The listing builds one solid part. Answer for the finished solid, in the listing's coordinates (mm). Face numbers are marked on the shaded views. A direction names the side the tool comes from. Coordinates: 2 decimals unless noted, no trailing zeros. Loops run counter-clockwise (first coordinate to the right, second up) from the corner with the lowest first, then second, coordinate; pieces in that order, holes last. Notation, with made-up numbers: M 11,61.5 L 50,61.5 A27 cw 50,79.5 Z; hole C -32,11.5 d11. An arc over 180 degrees is marked long. Answer as a JSON object with one key per item and string values. Group by question number.
1. Straight lines are drawn through the part: L1, parallel to Z at x = 18, y = -8.5; L2, parallel to Z at x = -9, y = 3; L3, parallel to X at y = 0.75, z = -3.5. For each, find the intervals that lie inside material, in ascending order.
2. A cutting plane is placed at D-D on z = -3.5. Give the vertices of the cut face in (x, y).
3. A cutting plane is placed at A-A on x = 41. Give the vertices of the cut face in (y, z), and give its area (3 significant figures).
4. A cutting plane is placed at C-C on y = -5.75. Give the vertices of the cut face in (x, z).
5. Determine the mould class of the marked faces 5, 6 and 7 for opening direction Y: released by +Y, released by -Y, zero draft, split by the parting line, or undercut.
6. A cutting plane is placed at B-B on z = 7.75. Give the vertices of the cut face in (x, y).
7. Given pin 1 (4 mm diameter, centred on y = -1.5, z = 11.5, fed in from +X); pin 2 (10 mm diameter, centred on x = -5, y = -6, fed in from -Z); pin 3 (9.5 mm diameter, centred on x = 38.5, y = -1.5, fed in from +Z); pin 4 (7 mm diameter, centred on x = 13.5, y = -5.5, fed in from +Z), each flat-ended and moving along its own axis, determine where each tip first touches the part or whether it passes through.
8. For the marked faces 1, 2, 3 and 4, determine the directions among +Z, -Z, +X, -X, +Y, -Y from which every point of the face is accessible in a straight line to the end or side of a thin tool.
from build123d import *

# Parameters (mm, degrees)
SALIENTE_EXTRUIR2_DEPTH = 3
CROQUIS2_R              = 2
SALIENTE_EXTRUIR3_DEPTH = 8
CROQUIS3_W              = 15
CROQUIS3_H              = 19.925925926
SALIENTE_EXTRUIR4_DEPTH = 10
CHAFL_N1_SIZE           = 4
CHAFL_N2_SIZE           = 1
CROQUIS4_R              = 4
SALIENTE_EXTRUIR5_DEPTH = 3
CROQUIS5_R              = 5
SALIENTE_EXTRUIR6_DEPTH = 2
CROQUIS6_R              = 4.259259259
CORTAR_EXTRUIR1_DEPTH   = 1
CHAFL_N3_SIZE           = 1


with BuildPart() as part:
    # Croquis1 → Saliente-Extruir2 (new body)
    with BuildSketch(Plane.XY):
        Polygon((-15.510753344, -3.296296296), (7.989246656, -14.222222222), (22.989246656, -14.222222222), (46.489246656, -3.296296296), (46.489246656, 5.703703704), (-15.510753344, 5.703703704), align=None)
    extrude(amount=SALIENTE_EXTRUIR2_DEPTH)

    # Croquis2 → Saliente-Extruir3 (add)
    with BuildSketch(Plane(origin=(0, 0, 0), x_dir=(-1, 0, 0), z_dir=(0, 0, -1))):
        with Locations(Location((-41.489246656, 0.703703704, 0), (0, 0, 180))):
            Circle(CROQUIS2_R)
        with Locations(Location((10.510753344, 0.703703704, 0), (0, 0, 180))):
            Circle(CROQUIS2_R)
    extrude(amount=SALIENTE_EXTRUIR3_DEPTH)

    # Croquis3 → Saliente-Extruir4 (add)
    with BuildSketch(Plane.XY.offset(3)):
        with Locations((15.489246656, -4.259259259)):
            Rectangle(CROQUIS3_W, CROQUIS3_H)
    extrude(amount=SALIENTE_EXTRUIR4_DEPTH)

    # Chaflán1
    chafl_n1_edges = [part.edges().sort_by_distance(p)[0] for p in [
        (15.489246656, -14.222222222, 13),
        (15.489246656, 5.703703704, 13),
    ]]
    chamfer(chafl_n1_edges, length=CHAFL_N1_SIZE)

    # Chaflán2
    chafl_n2_edges = [part.edges().sort_by_distance(p)[0] for p in [
        (7.989246656, -4.259259259, 13),
        (22.989246656, -4.259259259, 13),
    ]]
    chamfer(chafl_n2_edges, length=CHAFL_N2_SIZE)

    # Croquis4 → Saliente-Extruir5 (add)
    with BuildSketch(Plane.XY.offset(13)):
        with Locations((15.489246656, -4.259259259)):
            Circle(CROQUIS4_R)
    extrude(amount=SALIENTE_EXTRUIR5_DEPTH)

    # Croquis5 → Saliente-Extruir6 (add)
    with BuildSketch(Plane.XY.offset(16)):
        with Locations((15.489246656, -4.259259259)):
            Circle(CROQUIS5_R)
    extrude(amount=SALIENTE_EXTRUIR6_DEPTH)

    # Croquis6 → Cortar-Extruir1 (cut)
    with BuildSketch(Plane.XY.offset(18)):
        with Locations((15.489246656, -4.259259259)):
            Circle(CROQUIS6_R)
    extrude(amount=-CORTAR_EXTRUIR1_DEPTH, mode=Mode.SUBTRACT)

    # Chaflán3
    chafl_n3_edges = [part.edges().sort_by_distance(p)[0] for p in [
        (34.739246656, 5.703703704, 3),
        (-3.760753344, 5.703703704, 3),
    ]]
    chamfer(chafl_n3_edges, length=CHAFL_N3_SIZE)


solid = part.part
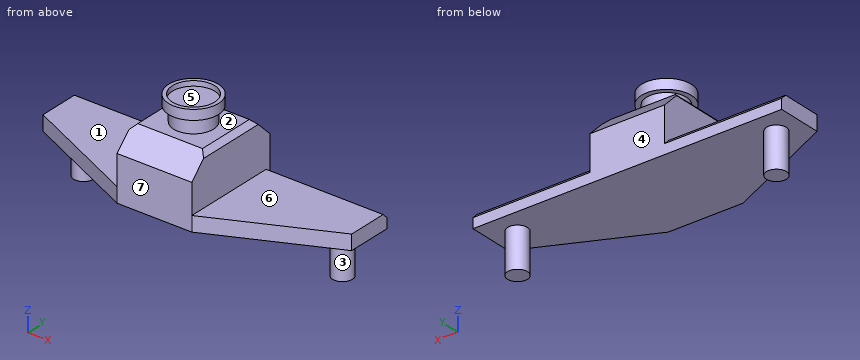
From the geometry:
{
 "1": {"L1": "z = 0 to 13, 16 to 18", "L2": "z = 0 to 3", "L3": "x = -12.51 to -8.51, 39.49 to 43.49"},
 "2": {"outline": "C -10.51,0.7 d4; C 41.49,0.7 d4"},
 "3": {"outline": "M -5.85,0 L -1.24,0 L -1.24,-8 L 2.64,-8 L 2.64,0 L 5.7,0 L 5.7,2 L 4.7,3 L -5.85,3 Z", "area": "65.2 mm²"},
 "4": {"outline": "M -10.23,0 L 41.21,0 L 41.21,3 L 22.99,3 L 22.99,12 L 21.99,13 L 19.2,13 L 19.2,16 L 20.26,16 L 20.26,18 L 19.48,18 L 19.48,17 L 11.5,17 L 11.5,18 L 10.72,18 L 10.72,16 L 11.78,16 L 11.78,13 L 8.99,13 L 7.99,12 L 7.99,3 L -10.23,3 Z"},
 "5": {"face 5": "undercut", "face 6": "zero draft", "face 7": "released by -Y"},
 "6": {"outline": "M 7.99,-14.22 L 22.99,-14.22 L 22.99,5.7 L 7.99,5.7 Z"},
 "7": {"pin 1": "stops at x = 22.99", "pin 2": "stops at z = 0", "pin 3": "stops at z = 3", "pin 4": "stops at z = 18"},
 "8": {"face 1": "+Z, -X, +Y, -Y", "face 2": "none", "face 3": "-Z", "face 4": "+Z, -Z, +X, -X, +Y"}
}
